```python
from build123d import *

# Parameters (mm, degrees)
F0_R     = 1.75
F0_R_2   = 1.5
F1_DEPTH = 6
F3_DEPTH = 6.001
F4_R     = 2


with BuildPart() as f1:
    # F0 (on Top) → F1 (new body)
    with BuildSketch(Plane.XY):
        with BuildLine():
            ThreePointArc((0, 40), (-20, 20), (0, 0))
            Line((0, 0), (205, 0))
            ThreePointArc((205, 0), (225, 20), (205, 40))
            Line((205, 40), (0, 40))
        make_face()
        with Locations((0, 5)):
            Circle(F0_R, mode=Mode.SUBTRACT)
        with Locations((-10.6066017178, 9.3933982822)):
            Circle(F0_R_2, mode=Mode.SUBTRACT)
        with Locations((10.6066017178, 9.3933982822)):
            Circle(F0_R_2, mode=Mode.SUBTRACT)
        with Locations((205, 5)):
            Circle(F0_R, mode=Mode.SUBTRACT)
        with Locations((215.6066017178, 9.3933982822)):
            Circle(F0_R_2, mode=Mode.SUBTRACT)
        with Locations((-15, 20)):
            Circle(F0_R, mode=Mode.SUBTRACT)
        with BuildLine():
            ThreePointArc((4, 20), (-3.69551813, 18.4692662705), (2.8284271247, 22.8284271247))
            ThreePointArc((2.8284271247, 22.8284271247), (3.69551813, 21.5307337295), (4, 20))
        make_face(mode=Mode.SUBTRACT)
        with Locations((15, 20)):
            Circle(F0_R, mode=Mode.SUBTRACT)
        with Locations((-10.6066017178, 30.6066017178)):
            Circle(F0_R_2, mode=Mode.SUBTRACT)
        with BuildLine():
            ThreePointArc((12.1066017178, 30.6066017178), (11.1806268663, 29.220782419), (9.545941546, 29.545941546))
            ThreePointArc((9.545941546, 29.545941546), (10.0325765693, 31.9924210166), (12.1066017178, 30.6066017178))
        make_face(mode=Mode.SUBTRACT)
        with Locations((0, 35)):
            Circle(F0_R, mode=Mode.SUBTRACT)
        with Locations((215.6066017178, 30.6066017178)):
            Circle(F0_R_2, mode=Mode.SUBTRACT)
        with Locations((205, 35)):
            Circle(F0_R, mode=Mode.SUBTRACT)
    extrude(amount=F1_DEPTH)

    # F2 (on face) → F3 (cut, through all)
    with BuildSketch(Plane.XY.offset(6)):
        Polygon((55.0816150746, 34), (22.75, 34), (38.9158075373, 6), align=None)
        Polygon((62.0098183049, 34), (45.8440107676, 6), (78.1756258422, 6), align=None)
        Polygon((85.1038290725, 6), (101.2696366098, 34), (68.9380215352, 34), align=None)
        Polygon((124.3636473774, 6), (108.1978398401, 34), (92.0320323028, 6), align=None)
        Polygon((131.2918506076, 6), (147.457658145, 34), (115.1260430703, 34), align=None)
        Polygon((170.5516689125, 6), (154.3858613752, 34), (138.2200538379, 6), align=None)
        Polygon((177.4798721428, 6), (193.6456796801, 34), (161.3140646055, 34), align=None)
        Polygon((200.5738829104, 6), (200.5738829104, 34), (184.4080753731, 6), align=None)
        Polygon((22.75, 22), (22.75, 6), (31.987604307, 6), align=None)
    extrude(amount=-F3_DEPTH, mode=Mode.SUBTRACT)

    # F4
    f4_edges = [f1.edges().sort_by_distance(p)[0] for p in [
        (22.75, 34, 3),
        (55.081615, 34, 3),
        (38.915808, 6, 3),
        (45.844011, 6, 3),
        (62.009818, 34, 3),
        (78.175626, 6, 3),
        (22.75, 22, 3),
        (22.75, 6, 3),
        (31.987604, 6, 3),
        (68.938022, 34, 3),
        (101.269637, 34, 3),
        (85.103829, 6, 3),
        (92.032032, 6, 3),
        (108.19784, 34, 3),
        (124.363647, 6, 3),
        (115.126043, 34, 3),
        (161.314065, 34, 3),
        (147.457658, 34, 3),
        (193.64568, 34, 3),
        (131.291851, 6, 3),
        (154.385861, 34, 3),
        (170.551669, 6, 3),
        (138.220054, 6, 3),
        (200.573883, 6, 3),
        (184.408075, 6, 3),
        (200.573883, 34, 3),
    ]]
    fillet(f4_edges, radius=F4_R)


solid = f1.part
```
Source: CAD feature listing. Evaluate the final solid. Frame: model axes, mm. A direction names the side the tool comes from. Give positions to 0.01 mm unless a question says otherwise; leave off trailing zeros.
1. Access query for faces 1 (the face through (-20, 20, 3)), 2 (the face through (27, 6, 3)). Directions: +Z, -Z, +X, -X, +Y, -Y. A direction counts if a zero-diameter tool reaches every point of the face in a straight line with its end or side. Return the directions, or none.
2. Pull-direction query (X, two-part tool) for faces 3 (the face through (101, 25, 6)), 4 (the face through (225, 20, 3)), 5 (the face through (62, 6, 3)); classes: +X half, -X half, draft (parallel to the pull), parting line (faces both ways), or undercut.
3. Material intervals for line 1 along Y through (x, z) = (205, 2.65); line 2 along Y through (x, z) = (119, 5.25); line 3 along Y through (x, z) = (131, 2.75), sorted ascending.
4. Section query A-A (z = 4.25). Count the separate pieces of the cut face and the enclosed holes in it, then the cut area to 3 significant figures.
5. First-contact query: pin 1 (3 mm diameter, centred on y = 33, z = 2.5, fed in from -X); pin 2 (1.8 mm diameter, centred on y = 11, z = 2, fed in from +X); pin 3 (2 mm diameter, centred on y = 23, z = 2.5, fed in from +X). Flat tips, straight axial feed; report the tip coordinate or a pass-through.
Output values:
1. face 1: +Z, -Z, -X
1. face 2: +Z, -Z
2. face 3: draft
2. face 4: +X half
2. face 5: undercut
3. line 1: y = 0 to 3.25, 6.75 to 33.25, 36.75 to 40
3. line 2: y = 0 to 6, 15.29 to 27.29, 34 to 40
3. line 3: y = 0 to 8.02, 34 to 40
4. separate pieces: 1
4. enclosed holes: 22
4. area: 5,920 mm2
5. pin 1: stops at x = -16.36
5. pin 2: stops at x = 223.29
5. pin 3: stops at x = 224.9
